Answer from the drawing. Dimensions are ordinates in mm from the lowest x, y and z of the part. Round coordinates to 2 decimals unless told otherwise and drop trailing zeros. Loops run counter-clockwise (first coordinate to the right, second up) from the corner with the lowest first, then second, coordinate; pieces in that order, holes last.
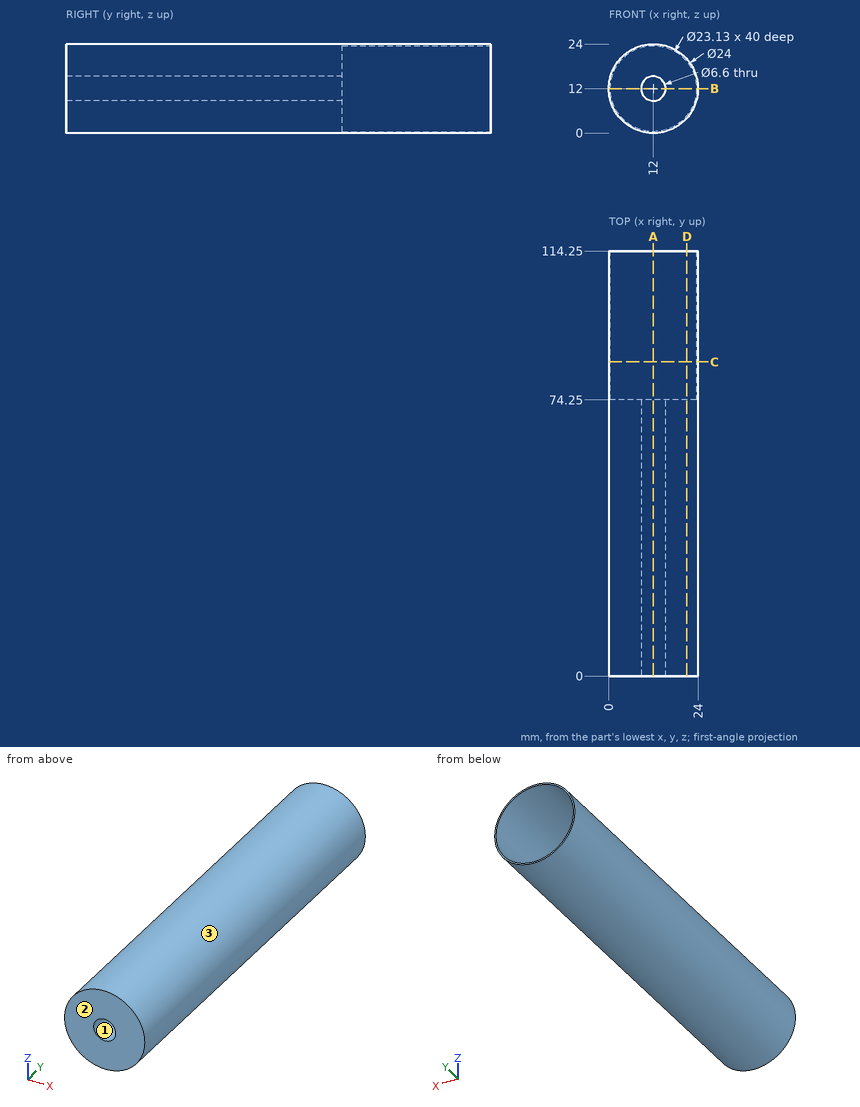
1. Consider probe 1 along Z at (x, y) = (12, 97) (3 decimals); probe 2 along Z at (x, y) = (12, 19.5). Determine where each line is inside the solid, lowest interval first.
Answer key:
probe 1: z = 0 to 0.435, 23.565 to 24
probe 2: z = 0 to 8.7, 15.3 to 24
2. Find section C-C (y = 84.5). Write down the section's boundary in (x, z) (3 decimals), then the cut area to 3 significant figures.
Answer key:
outline: circle Ø24 at (12, 12); hole circle Ø23.13 at (12, 12)
area: 32.2 mm2
3. Find section B-B (z = 12). Write down the section's boundary in (x, y) (3 decimals).
Answer key:
outline: (0, 0) - (8.7, 0) - (8.7, 74.25) - (0.435, 74.25) - (0.435, 114.25) - (0, 114.25) - close; (15.3, 0) - (24, 0) - (24, 114.25) - (23.565, 114.25) - (23.565, 74.25) - (15.3, 74.25) - close
4. Find section D-D (x = 21). Write down the section's boundary in (y, z), then the cut area to 3 significant figures.
Answer key:
outline: (0, 4.06) - (114.25, 4.06) - (114.25, 4.74) - (74.25, 4.74) - (74.25, 19.26) - (114.25, 19.26) - (114.25, 19.94) - (0, 19.94) - close
area: 1,230 mm2
5. Find section A-A (x = 12). Write down the section's boundary in (y, z) (3 decimals), then the cut area to 3 significant figures.
Answer key:
outline: (0, 0) - (114.25, 0) - (114.25, 0.435) - (74.25, 0.435) - (74.25, 8.7) - (0, 8.7) - close; (0, 15.3) - (74.25, 15.3) - (74.25, 23.565) - (114.25, 23.565) - (114.25, 24) - (0, 24) - close
area: 1,330 mm2
6. Determine the mould class of the marked faces 1, 2 and 3 for opening direction X: +X half, -X half, draft (parallel to the pull), parting line (faces both ways), or undercut.
Answer key:
face 1: undercut
face 2: draft
face 3: parting line
7. Given pin 1 (6 mm diameter, centred on x = 8.5, z = 11.5, fed in from +Y); pin 2 (6 mm diameter, centred on x = 17, y = 51, fed in from +Z); pin 3 (2 mm diameter, centred on x = 4, y = 29.5, fed in from -Z), each flat-ended and moving along its own axis, determine where each tip first touches the part or whether it passes through.
Answer key:
pin 1: stops at y = 74.25
pin 2: stops at z = 23.83
pin 3: stops at z = 2.25
